```python
from build123d import *

# Parameters (mm, degrees)
SKETCH2_W           = 11.7856
SKETCH2_H           = 11.7856
BOSS_EXTRUDE1_DEPTH = 0.635
BOSS_EXTRUDE2_DEPTH = 0.635
BOSS_EXTRUDE3_DEPTH = 1.4478
BOSS_EXTRUDE4_DEPTH = 11.5443
SKETCH6_R           = 1.09855
BOSS_EXTRUDE5_DEPTH = 0.9779
SKETCH7_W           = 1.509743552
SKETCH7_H           = 1.27
CUT_EXTRUDE1_DEPTH  = 14.0843


with BuildPart() as part:
    # Sketch1 → Revolve1 (revolve)
    with BuildSketch(Plane.XY):
        Polygon((0, 0), (5.925, 0), (5.925, 14.0843), (3.75, 14.0843), (3.75, 19.8755), (4.36245, 19.8755), (4.36245, 25.3365), (0, 25.3365), align=None)
    revolve(axis=Axis((0, 31.195966839, 0), (0, -1, 0)))

    # Sketch2 → Boss-Extrude1 (add)
    with BuildSketch(Plane.XZ):
        Rectangle(SKETCH2_W, SKETCH2_H)
    extrude(amount=BOSS_EXTRUDE1_DEPTH)

    # Sketch3 → Boss-Extrude2 (add)
    with BuildSketch(Plane.XZ.offset(0.635)):
        with BuildLine():
            Line((-3.98145, 6.33095), (12.6492, 6.33095))
            Line((12.6492, 6.33095), (12.6492, -6.33095))
            Line((12.6492, -6.33095), (-3.98145, -6.33095))
            ThreePointArc((-3.98145, -6.33095), (-10.3124, 0), (-3.98145, 6.33095))
        make_face()
    extrude(amount=BOSS_EXTRUDE2_DEPTH)

    # Sketch4 → Boss-Extrude3 (add)
    with BuildSketch(Plane.XZ.offset(1.27)):
        with BuildLine():
            Line((-3.98145, -6.33095), (15.1892, -6.33095))
            Line((15.1892, -6.33095), (15.1892, 6.33095))
            Line((15.1892, 6.33095), (-3.98145, 6.33095))
            ThreePointArc((-3.98145, 6.33095), (-10.3124, 0), (-3.98145, -6.33095))
        make_face()
    extrude(amount=BOSS_EXTRUDE3_DEPTH)

    # Sketch5 → Boss-Extrude4 (add)
    with BuildSketch(Plane.XZ.offset(2.7178)):
        with BuildLine():
            Line((12.0396, 6.33095), (-3.98145, 6.33095))
            ThreePointArc((-3.98145, 6.33095), (-10.3124, 0), (-3.98145, -6.33095))
            Line((-3.98145, -6.33095), (12.0396, -6.33095))
            Line((12.0396, -6.33095), (12.0396, 6.33095))
        make_face()
    extrude(amount=BOSS_EXTRUDE4_DEPTH)

    # Sketch6 → Boss-Extrude5 (add)
    with BuildSketch(Plane.XY.offset(3.33375)):
        with BuildLine():
            Line((14.097, -8.4074), (14.097, -11.5062))
            Line((14.097, -11.5062), (12.0396, -11.5062))
            Line((12.0396, -11.5062), (12.0396, -2.7178))
            Line((12.0396, -2.7178), (14.097, -2.7178))
            Line((14.097, -2.7178), (14.097, -5.8166))
            Line((14.097, -5.8166), (14.890270235, -5.8166))
            ThreePointArc((14.890270235, -5.8166), (19.2278, -7.112), (14.890270235, -8.4074))
            Line((14.890270235, -8.4074), (14.097, -8.4074))
        make_face()
        with Locations((16.8656, -7.112)):
            Circle(SKETCH6_R, mode=Mode.SUBTRACT)
    boss_extrude5 = extrude(amount=-BOSS_EXTRUDE5_DEPTH)

    # Mirror1: Boss-Extrude5 across plane
    add(boss_extrude5.mirror(Plane.XY))

    # Sketch7 → Cut-Extrude1 (cut)
    with BuildSketch(Plane(origin=(0, 14.0843, 0), x_dir=(1, 0, 0), z_dir=(0, 1, 0))):
        with Locations((6.070418397, 0)):
            Rectangle(SKETCH7_W, SKETCH7_H)
    extrude(amount=-CUT_EXTRUDE1_DEPTH, mode=Mode.SUBTRACT)


solid = part.part
```
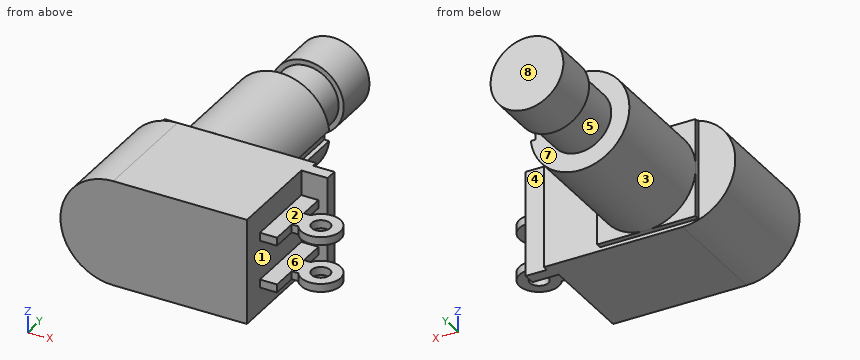
Model file for the job. Use its own axes, mm. Face numbers are marked on the shaded views. A direction names the side the tool comes from. Round coordinates to 2 decimals unless told otherwise and drop trailing zeros. Loops run counter-clockwise (first coordinate to the right, second up) from the corner with the lowest first, then second, coordinate; pieces in that order, holes last. Notation, with made-up numbers: M 86,-11 L 137,-11 A23 ccw 137,-3 Z; hole C 60,-38 d10. An arc over 180 degrees is marked long. Put each result on its own line as item: value. Start each with the question number.
Item 1: Cut at D-D (y = -2). List the corners of the cut face in (x, z).
Item 2: Cut at A-A (y = -9). List the corners of the cut face in (x, z).
Item 3: Mould opens along Y. For the marked faces 5, 6, 7 and 8 say: released by +Y, released by -Y, zero draft, split by the parting line, or undercut.
Item 4: Drop flat-ended pins along their axis: P1, Ø0.6, axis at x = 14.5, z = 2.5, coming from the -Y side; P2, Ø1.5, axis at x = -6, y = -3, coming from the +Z side; P3, Ø0.8, axis at x = 13, z = -3, coming from the -Y side. Give the stop position or say it passes through.
Item 5: 3-axis set-ups, long thin cutter, end or side, ignore diameter. For the marked faces 1, 2, 3 and 4: which of +Z, -Z, +X, -X, +Y, -Y reach the whole face in a straight line?
Item 6: Drill centre lines: line 1 along Y through (x, z) = (1.75, -4.5); line 2 along X through (y, z) = (13.5, 0.25); line 3 along Y through (x, z) = (13.25, -0.5). Where is each one in solid material? Low to high.
Answer block:
1. outline: M -3.98,-6.33 L 15.19,-6.33 L 15.19,6.33 L -3.98,6.33 A6.33 ccw Z
2. outline: M -3.98,-6.33 L 12.04,-6.33 L 12.04,-3.33 L 14.1,-3.33 L 14.1,-2.36 L 12.04,-2.36 L 12.04,2.36 L 14.1,2.36 L 14.1,3.33 L 12.04,3.33 L 12.04,6.33 L -3.98,6.33 A6.33 ccw Z; M 15.45,-3.33 L 18.29,-3.33 L 18.29,-2.36 L 15.45,-2.36 Z; M 15.45,2.36 L 18.29,2.36 L 18.29,3.33 L 15.45,3.33 Z
3. face 5: undercut
3. face 6: zero draft
3. face 7: undercut
3. face 8: released by +Y
4. P1: y = -8.41
4. P2: z = 6.2
4. P3: y = -11.51
5. face 1: +X, -Y
5. face 2: +Z, +X, -Y
5. face 3: +Y
5. face 4: +Z, -Z, +X, +Y
6. line 1: -14.26 to 14.08
6. line 2: -5.92 to 5.32
6. line 3: -2.72 to -1.27
